Verification items for this drawing (mm, ordinates from the low corner). A direction names the side the tool comes from. Round coordinates to 2 decimals unless told otherwise and drop trailing zeros. Loops run counter-clockwise (first coordinate to the right, second up) from the corner with the lowest first, then second, coordinate; pieces in that order, holes last. Notation, with made-up numbers: M -11.5,17.25 L 14.5,17.25 A22 cw 14.5,52.25 Z; hole C 60,42.5 d4. An arc over 180 degrees is marked long. One line per item, written item: value.
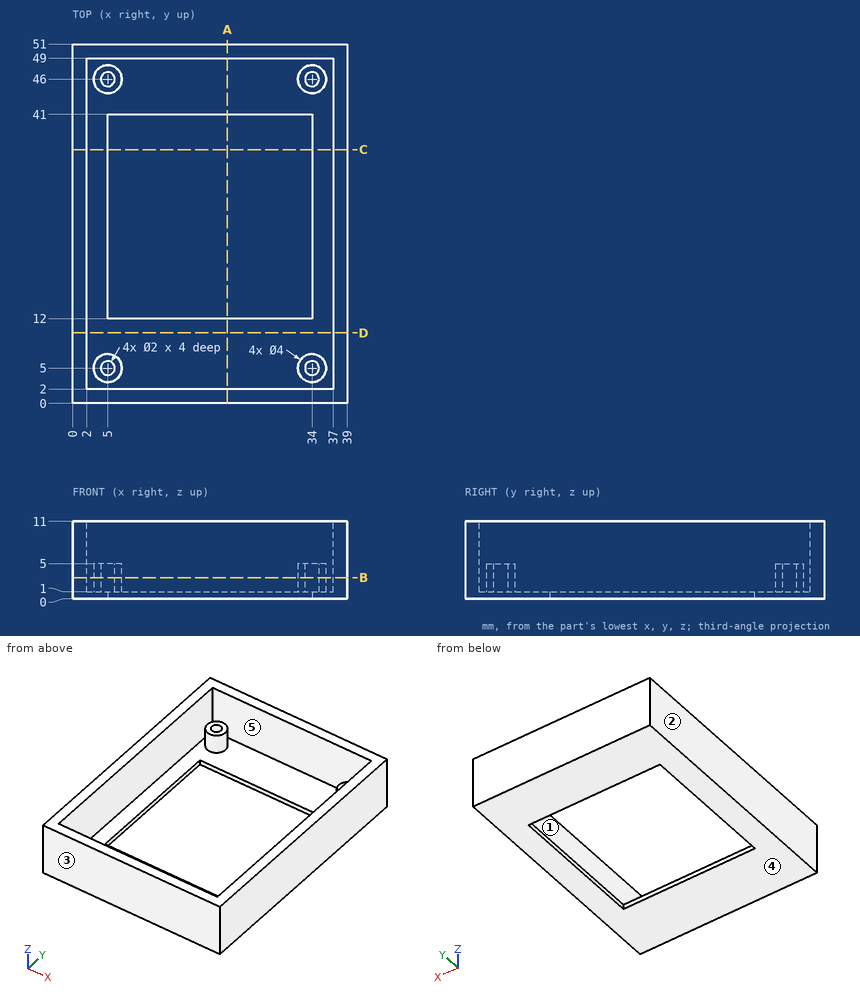
(1) Sectioned sample at A-A on x = 22. Enter the section's corners in (y, z), and give its area (3 significant figures).
Completed:
outline: M 0,0 L 12,0 L 12,1 L 2,1 L 2,11 L 0,11 Z; M 41,0 L 51,0 L 51,11 L 49,11 L 49,1 L 41,1 Z
area: 62.0 mm^2
(2) Sectioned sample at B-B on z = 3. Count the separate pieces of the cut face and the enclosed holes in it, and give its area (3 significant figures).
Completed:
separate pieces: 5
enclosed holes: 5
area: 382 mm^2
(3) Thickness scan on L1, parallel to Y at x = 34, z = 3.9; L2, parallel to X at y = 45.5, z = 5.5; L3, parallel to Y at x = 25.5, z = 1.75. Record the ranges inside material, lowest first. Write a range as from..to.
Completed:
L1: y = 0..2, 3..4, 6..7, 44..45, 47..48, 49..51
L2: x = 0..2, 37..39
L3: y = 0..2, 49..51
(4) Tool access check on the marked faces 4 and 5. Record the directions out of +Z, -Z, +X, -X, +Y, -Y that give a thin tool (end or side, any length) a straight path to the whole face; none if there is none.
Completed:
face 4: -Z, +X, -X, +Y, -Y
face 5: +Z
(5) Sectioned sample at D-D on y = 10. Enter the section's corners in (x, z).
Completed:
outline: M 0,0 L 39,0 L 39,11 L 37,11 L 37,1 L 2,1 L 2,11 L 0,11 Z
(6) Mould release check, pull along Y, two halves, no side actions. Record for the marked faces 1, 2 and 3: +Y half, -Y half, draft (parallel to the pull), parting line (faces both ways), or undercut.
Completed:
face 1: undercut
face 2: draft
face 3: -Y half
(7) Sectioned sample at C-C on y = 36. Enter the section's corners in (x, z).
Completed:
outline: M 0,0 L 5,0 L 5,1 L 2,1 L 2,11 L 0,11 Z; M 34,0 L 39,0 L 39,11 L 37,11 L 37,1 L 34,1 Z
(8) Depth check by flat-ended pin: pin 1 Ø1.6 at (x, y) = (5, 46) entering from +Z; pin 2 Ø3 at (x, y) = (34.5, 46.5) entering from +Z; pin 3 Ø8 at (x, y) = (28.5, 29.5) entering from -Z. Enter the tip coordinate at first touch or a pass-through.
Completed:
pin 1: stops at z = 1
pin 2: stops at z = 5
pin 3: passes through
